from build123d import *

# Parameters (mm, degrees)
SKETCH_1_R      = 20
EXTRUDE_1_DEPTH = 6


with BuildPart() as part:
    # 草图1 → 拉伸1 (new body)
    with BuildSketch(Plane.XY):
        with BuildLine():
            Line((34.379807383, -3), (37.379807383, -3))
            ThreePointArc((37.379807383, -3), (26.516504294, -26.516504294), (3, -37.379807383))
            Line((3, -37.379807383), (3, -34.379807383))
            Line((3, -34.379807383), (-3, -34.379807383))
            Line((-3, -34.379807383), (-3, -37.379807383))
            ThreePointArc((-3, -37.379807383), (-26.516504294, -26.516504294), (-37.379807383, -3))
            Line((-37.379807383, -3), (-34.379807383, -3))
            Line((-34.379807383, -3), (-34.379807383, 3))
            Line((-34.379807383, 3), (-37.379807383, 3))
            ThreePointArc((-37.379807383, 3), (-26.516504294, 26.516504294), (-3, 37.379807383))
            Line((-3, 37.379807383), (-3, 34.379807383))
            Line((-3, 34.379807383), (3, 34.379807383))
            Line((3, 34.379807383), (3, 37.379807383))
            ThreePointArc((3, 37.379807383), (26.516504294, 26.516504294), (37.379807383, 3))
            Line((37.379807383, 3), (34.379807383, 3))
            Line((34.379807383, 3), (34.379807383, -3))
        make_face()
        Circle(SKETCH_1_R, mode=Mode.SUBTRACT)
    extrude(amount=EXTRUDE_1_DEPTH)


solid = part.part
Could you check a few things on this model? Use its own coordinates, in mm. A direction names the side the tool comes from. Coordinates: 2 decimals unless noted, no trailing zeros. Order: outer loops, then holes, each group sorted by start corner. A loop starts at its lowest first (then second) coordinate and runs counter-clockwise, first axis right, second up.
Q1. Please list where these lines run through material, in increasing order: L1, parallel to Y at x = 0, z = 3.2; L2, parallel to Y at x = -2, z = 3.7; L3, parallel to X at y = -6.5, z = 1.6.
Q2. Suppose I cut it at A-A on x = 0. Please give me the cut outline in (y, z).
Q3. Thinking about a two-plate mould opening in X: for faces 1 (the flat face through (-3, 36, 3)), 2 (the flat face through (0, 34.38, 3)), 3 (the flat face through (-36, 3, 3)), 4 (the flat face through (-34.38, 0, 3)), which applies, released by +X, released by -X, zero draft, split by the parting line, or undercut?
Q4. Will these pins go through, and if not, where does the flat tip stop? pin 1 (1.5 mm diameter, centred on y = -35, z = 1.5, fed in from +X); pin 2 (1.5 mm diameter, centred on y = -14.5, z = 3, fed in from +X); pin 3 (3 mm diameter, centred on x = 0, z = 3.5, fed in from -Y); pin 4 (3 mm diameter, centred on x = 14, y = -27, fed in from -Z).
Q5. Which directions (+Z, -Z, +X, -X, +Y, -Y) give clear straight access to the entire face, cutting with the end or side of a thin tool? Please do faces 5 (the flat face through (3, 36, 3)), 6 (the cylindrical face through (26.78, -26.25, 2.96)), 7 (the flat face through (-36, -3, 3)), 8 (the flat face through (36, 3, 3)), 9 (the flat face through (-3, -36, 3)).
Q6. Suppose I cut it at D-D on x = -21.5. Please give me the cut outline in (y, z), and give its area (3 significant figures).
Q7. Suppose I cut it at C-C on z = 4.25. Please give me the cut outline in (x, y).
Answer:
1. L1: y = -34.38 to -20, 20 to 34.38
1. L2: y = -34.38 to -19.9, 19.9 to 34.38
1. L3: x = -36.93 to -18.91, 18.91 to 36.93
2. outline: (-34.38, 0) - (-20, 0) - (-20, 6) - (-34.38, 6) - close; (20, 0) - (34.38, 0) - (34.38, 6) - (20, 6) - close
3. face 1: undercut
3. face 2: undercut
3. face 3: zero draft
3. face 4: released by -X
4. pin 1: stops at x = 15.27
4. pin 2: stops at x = 34.89
4. pin 3: stops at y = -34.38
4. pin 4: stops at z = 0
5. face 5: +Z, -Z, +Y
5. face 6: +Z, -Z, +X, -Y
5. face 7: +Z, -Z, -X
5. face 8: +Z, -Z, +X
5. face 9: +Z, -Z, -Y
6. outline: (-30.72, 0) - (30.72, 0) - (30.72, 6) - (-30.72, 6) - close
6. area: 369 mm2
7. outline: (-37.38, -3) arc R37.5 ccw to (-3, -37.38) - (-3, -34.38) - (3, -34.38) - (3, -37.38) arc R37.5 ccw to (37.38, -3) - (34.38, -3) - (34.38, 3) - (37.38, 3) arc R37.5 ccw to (3, 37.38) - (3, 34.38) - (-3, 34.38) - (-3, 37.38) arc R37.5 ccw to (-37.38, 3) - (-34.38, 3) - (-34.38, -3) - close; hole circle Ø40 at (0, 0)
